Could you check a few things on this model? Use its own coordinates, in mm. Face numbers are marked on the shaded views. Give positions to 0.01 mm unless a question says otherwise; leave off trailing zeros. Order: outer loops, then holes, each group sorted by start corner. A loop starts at its lowest first (then second) coordinate and runs counter-clockwise, first axis right, second up.
(1) If I drill on probe 1 along Y at (x, z) = (-3, 1.5); probe 2 along X at (y, z) = (0.25, 0.3); probe 3 along X at (y, z) = (-2.25, 1.5), over which ranges is the centre line in solid material (lowest first)?
(2) If we mould it in two halves opening along Y, with no side actions, what happens to the marked faces 1, 2 and 3? For each: released by +Y, released by -Y, zero draft, split by the parting line, or undercut.
(3) Imagine slicing it at B-B, the plane y = 1. Write out the boundary of the cut face in (x, z), then the cut area to 3 significant figures.
(4) Imagine slicing it at C-C, the plane z = 3.15. Write out the boundary of the cut face in (x, y), then the cut area to 3 significant figures.
(5) Imagine slicing it at D-D, the plane x = 3.25. Write out the boundary of the cut face in (y, z), then the cut area to 3 significant figures.
(6) Imagine slicing it at A-A, the plane x = 0. Write out the boundary of the cut face in (y, z), then the cut area to 3 significant figures.
from build123d import *

# Parameters (mm, degrees)
F0_W     = 10
F0_H     = 7
F1_DEPTH = 5
F3_DEPTH = 7
F5_R     = 3.5
F6_DEPTH = 0.7
F8_R     = 3.5
F9_DEPTH = 0.9


with BuildPart() as f1:
    # F0 (on Top) → F1 (new body)
    with BuildSketch(Plane.XY):
        Rectangle(F0_W, F0_H)
    extrude(amount=F1_DEPTH)

    # F2 (on face) → F3 (cut, through all)
    with BuildSketch(Plane(origin=(0, 3.5, 0), x_dir=(-1, 0, 0), z_dir=(0, 1, 0))):
        with BuildLine():
            Line((-2, 0), (2, 0))
            ThreePointArc((2, 0), (0, 2), (-2, 0))
        make_face()
    extrude(amount=-F3_DEPTH, mode=Mode.SUBTRACT)

    # F5 (on offset) → F6 (cut)
    with BuildSketch(Plane(origin=(0, 2, 0), x_dir=(-1, 0, 0), z_dir=(0, 1, 0))):
        Circle(F5_R)
    extrude(amount=-F6_DEPTH, mode=Mode.SUBTRACT)

    # F8 (on offset) → F9 (cut)
    with BuildSketch(Plane(origin=(0, -0.3, 0), x_dir=(-1, 0, 0), z_dir=(0, 1, 0))):
        Circle(F8_R)
    extrude(amount=-F9_DEPTH, mode=Mode.SUBTRACT)


solid = f1.part
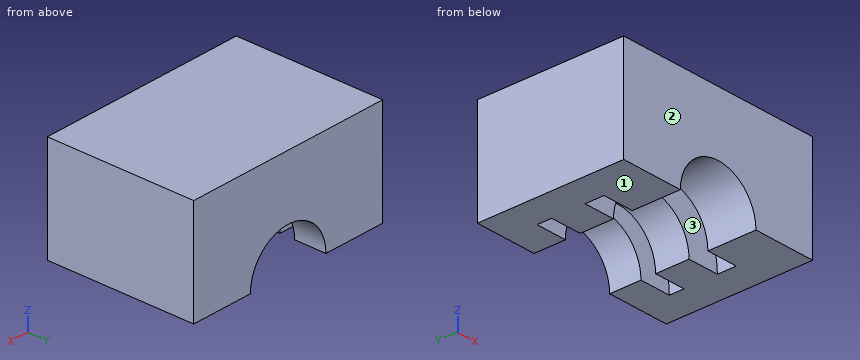
Answer block:
1. probe 1: y = -3.5 to -1.2, -0.3 to 1.3, 2 to 3.5
1. probe 2: x = -5 to -1.98, 1.98 to 5
1. probe 3: x = -5 to -1.32, 1.32 to 5
2. face 1: zero draft
2. face 2: released by -Y
2. face 3: undercut
3. outline: (-5, 0) - (-2, 0) arc R2 cw to (2, 0) - (5, 0) - (5, 5) - (-5, 5) - close
3. area: 43.7 mm2
4. outline: (-5, -3.5) - (5, -3.5) - (5, 3.5) - (-5, 3.5) - close; hole (-1.53, -1.2) - (1.53, -1.2) - (1.53, -0.3) - (-1.53, -0.3) - close; hole (-1.53, 1.3) - (1.53, 1.3) - (1.53, 2) - (-1.53, 2) - close
4. area: 65.1 mm2
5. outline: (-3.5, 0) - (-1.2, 0) - (-1.2, 1.3) - (-0.3, 1.3) - (-0.3, 0) - (1.3, 0) - (1.3, 1.3) - (2, 1.3) - (2, 0) - (3.5, 0) - (3.5, 5) - (-3.5, 5) - close
5. area: 32.9 mm2
6. outline: (-3.5, 2) - (-1.2, 2) - (-1.2, 3.5) - (-0.3, 3.5) - (-0.3, 2) - (1.3, 2) - (1.3, 3.5) - (2, 3.5) - (2, 2) - (3.5, 2) - (3.5, 5) - (-3.5, 5) - close
6. area: 18.6 mm2
